Read the model definition and answer for the solid it produces. Units are mm, in the model's axes. Face numbers are marked on the shaded views. A direction names the side the tool comes from. Round coordinates to 2 decimals unless told otherwise and drop trailing zeros. Order: outer loops, then holes, each group sorted by start corner. A loop starts at its lowest first (then second) coordinate and runs counter-clockwise, first axis right, second up. Notation, with made-up numbers: (-3.5, 37.25) - (36.5, 37.25) arc R18 cw to (36.5, 51.25) - close; hole circle Ø8 at (30.5, -17). An arc over 180 degrees is marked (long way). One line per question, with ' | ' between items. Start each with the question number.
1) The part is cut by section A-A, the plane y = 0. Give the vertices of the cut face in (x, z), plus the area to 3 significant figures.
2) The part is cut by section B-B, the plane x = 0. Give the vertices of the cut face in (y, z), plus the area to 3 significant figures.
3) For the marked faces 4 and 5, determine the directions among +Z, -Z, +X, -X, +Y, -Y from which every point of the face is accessible in a straight line to the end or side of a thin tool.
4) The mould has two halves that part along Z. Classify the marked faces 1, 2 and 3: pulls with the +Z half, pulls with the -Z half, needs draft (parallel to the pull), parting line crosses it, or undercut.
5) Flat-ended cylindrical pins translate along their axes: pin 1 (1 mm diameter, centred on x = 0.5, z = -0.5, fed in from -Y); pin 2 (3 mm diameter, centred on y = 1.5, z = -6, fed in from +X); pin 3 (2 mm diameter, centred on x = -2, z = -6.5, fed in from +Y). Find the tip coordinate at first contact, or state that the pin passes through.
6) The part is cut by section C-C, the plane z = 6.25. Give the vertices of the cut face in (x, y).
7) Straight lines are drawn through the part: line 1 (Z direction, x = 1.25, y = 3); line 2 (Z direction, x = 0.75, y = -0.25); line 3 (Y direction, x = 0.5, z = -8). For each, find the intervals that lie inside material, in ascending order. Write a range as from..to.
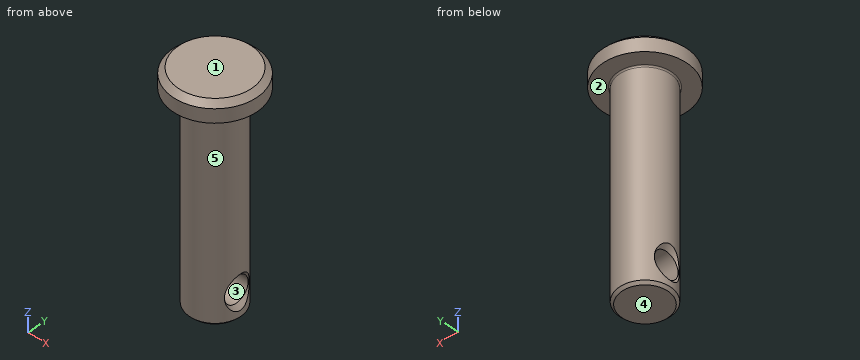
from build123d import *

# Parameters (mm, degrees)
CUT_EXTRUDE1_DEPTH      = 12.808951435
CUT_EXTRUDE1_DEPTH_BACK = 12.808951435
SKETCH3_R               = 1.1938


with BuildPart() as part:
    # Sketch2 → Revolve1 (revolve)
    with BuildSketch(Plane(origin=(0, 0, 0), x_dir=(0, 0, -1), z_dir=(1, 0, 0)), mode=Mode.PRIVATE) as revolve1_sk:
        with BuildLine():
            Line((10.17524, 2.3876), (-8.51662, 2.3876))
            ThreePointArc((-8.51662, 2.3876), (-8.601034408, 2.422565592), (-8.636, 2.50698))
            Line((-8.636, 2.50698), (-8.636, 3.937))
            Line((-8.636, 3.937), (-9.906, 3.937))
            Line((-9.906, 3.937), (-10.414, 3.429))
            Line((-10.414, 3.429), (-10.414, 0))
            Line((-10.414, 0), (10.414, 0))
            Line((10.414, 0), (10.414, 2.14884))
            Line((10.414, 2.14884), (10.17524, 2.3876))
        make_face()
    revolve(revolve1_sk.sketch.rotate(Axis((0, 0, 10.414), (0, 0, -1)), 90), axis=Axis((0, 0, 10.414), (0, 0, -1)))

    # Sketch3 → Cut-Extrude1 (cut, two sides: drawn at the far end of the back side and taken through both)
    with BuildSketch(Plane(origin=(0, 0, 0), x_dir=(0, 0, -1), z_dir=(1, 0, 0)).offset(-CUT_EXTRUDE1_DEPTH_BACK)):
        with Locations((8.0264, 0)):
            Circle(SKETCH3_R)
    extrude(amount=CUT_EXTRUDE1_DEPTH + CUT_EXTRUDE1_DEPTH_BACK, mode=Mode.SUBTRACT)

    # Sketch4 → Cut-Revolve1 (revolve, cut)
    with BuildSketch(Plane(origin=(0, 0, 0), x_dir=(1, 0, 0), z_dir=(0, 1, 0)), mode=Mode.PRIVATE) as cut_revolve1_sk:
        Polygon((2.3876, 6.434666667), (0.795866667, 8.0264), (2.3876, 8.0264), align=None)
        Polygon((-2.3876, 8.0264), (-2.3876, 6.434666667), (-0.795866667, 8.0264), align=None)
    revolve(cut_revolve1_sk.sketch.rotate(Axis((2.3876, 0, -8.0264), (-1, 0, 0)), 180), axis=Axis((2.3876, 0, -8.0264), (-1, 0, 0)), mode=Mode.SUBTRACT)


solid = part.part
Values:
1) outline: (-3.94, 8.64) - (-2.51, 8.64) arc R0.12 cw to (-2.39, 8.52) - (-2.39, -6.43) - (-1.99, -6.83) - (1.99, -6.83) - (2.39, -6.43) - (2.39, 8.52) arc R0.12 cw to (2.51, 8.64) - (3.94, 8.64) - (3.94, 9.91) - (3.43, 10.41) - (-3.43, 10.41) - (-3.94, 9.91) - close; (-2.39, -10.18) - (-2.15, -10.41) - (2.15, -10.41) - (2.39, -10.18) - (2.39, -9.62) - (1.99, -9.22) - (-1.99, -9.22) - (-2.39, -9.62) - close | area: 92.9 mm^2
2) outline: (-3.94, 8.64) - (-2.51, 8.64) arc R0.12 cw to (-2.39, 8.52) - (-2.39, -10.18) - (-2.15, -10.41) - (2.15, -10.41) - (2.39, -10.18) - (2.39, 8.52) arc R0.12 cw to (2.51, 8.64) - (3.94, 8.64) - (3.94, 9.91) - (3.43, 10.41) - (-3.43, 10.41) - (-3.94, 9.91) - close; hole circle Ø2.39 at (0, -8.03) | area: 100 mm^2
3) face 4: -Z, +X, -X, +Y, -Y | face 5: -Z
4) face 1: pulls with the +Z half | face 2: pulls with the -Z half | face 3: undercut
5) pin 1: stops at y = -2.39 | pin 2: stops at x = 2.39 | pin 3: stops at y = 2.17
6) outline: circle Ø4.78 at (0, 0)
7) line 1: z = 8.64..10.41 | line 2: z = -10.41..-9.19, -6.86..10.41 | line 3: y = -2.33..-1.19, 1.19..2.33
